Here's how the part is built. I have some questions about the finished solid (model axes, mm). Face numbers are marked on the shaded views. Round coordinates to 2 decimals unless told otherwise and drop trailing zeros. Order: outer loops, then holes, each group sorted by start corner. A loop starts at its lowest first (then second) coordinate and runs counter-clockwise, first axis right, second up. Notation, with made-up numbers: M 39.5,39.25 L 69.5,39.25 A12 ccw 69.5,46.25 Z; hole C 25,46.5 d3. An arc over 180 degrees is marked long. Write item = value, one per line. Start each with the question number.
Item 1: I want a section at C-C, the plane z = 33.5. List the corners of the cut face in (x, y) for me.
Item 2: We'd pull the mould along X, two halves only. Please class the marked faces 1, 2 and 3: pulls with the +X half, pulls with the -X half, needs draft (parallel to the pull), parting line crosses it, or undercut.
Item 3: I want a section at D-D, the plane y = -28.5. List the corners of the cut face in (x, z) for me.
Item 4: I'm going to push flat-ended pins straight in: P1, Ø3, axis at x = -6.5, z = 56, coming from the -Y side; P2, Ø8, axis at x = -5, z = 37, coming from the +Y side. Where does each tip first touch, or does it pass through?
Item 5: Please list where these lines run through material, in increasing order: L1, parallel to Z at x = 5, y = -30; L2, parallel to X at y = 4, z = 56; L3, parallel to Y at x = 10, z = 48.
Item 6: I want a section at B-B, the plane y = 0. List the corners of the cut face in (x, z) for me, plus the area to 3 significant figures.
Item 7: I want a section at A-A, the plane x = 0. List the corners of the cut face in (y, z) for me, plus the area to 3 significant figures.
```python
from build123d import *

# Parameters (mm, degrees)
F0_W     = 72.5571736693
F0_H     = 51.1083565652
F1_DEPTH = 27.94
F2_R     = 19.4094724008
F3_DEPTH = 50.546
F4_DEPTH = 25.4


with BuildPart() as f1:
    # F0 (on Front) → F1 (new body, symmetric)
    with BuildSketch(Plane.XZ):
        Rectangle(F0_W, F0_H)
    extrude(amount=F1_DEPTH, both=True)

    # F2 (on face) → F3 (join, symmetric)
    with BuildSketch(Plane.XY.offset(25.5541782826)):
        Circle(F2_R)
    extrude(amount=F3_DEPTH, both=True)

    # F4 (add): a face of the model
    f4_faces = [f1.faces().sort_by_distance(p)[0] for p in [
        (0, -27.94, 0),
    ]]
    extrude(f4_faces, amount=F4_DEPTH)


solid = f1.part
```
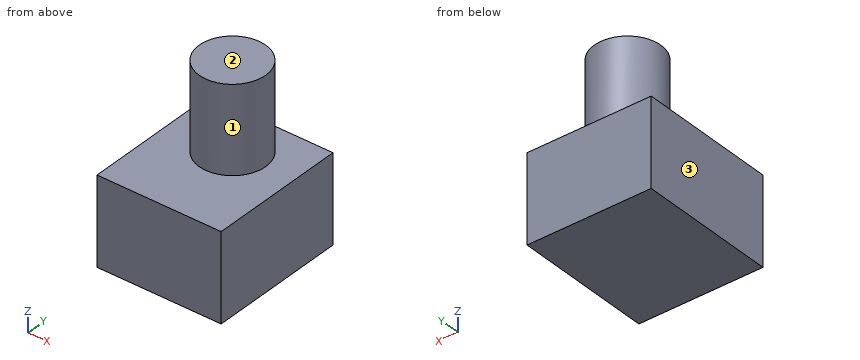
Filled in:
q1.outline = C 0,0 d38.82
q2.face_1 = parting line crosses it
q2.face_2 = needs draft
q2.face_3 = pulls with the -X half
q3.outline = M -36.28,-25.55 L 36.28,-25.55 L 36.28,25.55 L -36.28,25.55 Z
q4.P1 = -18.75
q4.P2 = 19.38
q5.L1 = -25.55 to 25.55
q5.L2 = -18.99 to 18.99
q5.L3 = -16.64 to 16.64
q6.outline = M -36.28,-25.55 L 36.28,-25.55 L 36.28,25.55 L 19.41,25.55 L 19.41,76.1 L -19.41,76.1 L -19.41,25.55 L -36.28,25.55 Z
q6.area = 5,670 mm^2
q7.outline = M -53.34,-25.55 L 27.94,-25.55 L 27.94,25.55 L 19.41,25.55 L 19.41,76.1 L -19.41,76.1 L -19.41,25.55 L -53.34,25.55 Z
q7.area = 6,120 mm^2
